```python
from build123d import *

# Parameters (mm, degrees)
SKETCH_1_W                         = 72
SKETCH_1_H                         = 40
EXTRUDE_1_DEPTH                    = 2
SKETCH_2_R                         = 7
CUT_EXTRUDE_1_DEPTH                = 3
FILLET_1_R                         = 3
SKETCH_5_R                         = 1.75
CUT_EXTRUDE_4_DEPTH                = 3
PATTERN_LINEAR_1_COUNT             = 2
PATTERN_LINEAR_1_PITCH             = 65
PATTERN_LINEAR_1_COUNT_DIR2        = 2
PATTERN_LINEAR_1_PITCH_DIR2        = 24
SKETCH_7_R                         = 2
SKETCH_7_R_2                       = 0.85
EXTRUDE_2_DEPTH                    = 3
SKETCH_8_R                         = 0.85
CUT_EXTRUDE_6_DEPTH                = 6
FILLET_3_R                         = 1
CHAMFER_1_SIZE                     = 0.6
PATTERN_LINEAR_2_COUNT             = 2
PATTERN_LINEAR_2_PITCH             = 12.5
PATTERN_LINEAR_2_COUNT_DIR2        = 2
PATTERN_LINEAR_2_PITCH_DIR2        = 21
FILLET_3_OF_PATTERN_LINEAR_2_R     = 1
CHAMFER_1_OF_PATTERN_LINEAR_2_SIZE = 0.6
CHAMFER_2_SIZE                     = 0.3


with BuildPart() as part:
    # Эскиз1 → Бобышка-Вытянуть1 (new body)
    with BuildSketch(Plane.XY):
        Rectangle(SKETCH_1_W, SKETCH_1_H)
    extrude(amount=EXTRUDE_1_DEPTH)

    # Эскиз2 → Вырез-Вытянуть1 (cut, through all)
    with BuildSketch(Plane.XY.offset(2)):
        Circle(SKETCH_2_R)
    extrude(amount=-CUT_EXTRUDE_1_DEPTH, mode=Mode.SUBTRACT)

    # Скругление1
    fillet_1_edges = [part.edges().sort_by_distance(p)[0] for p in [
        (36, -20, 1),
        (-36, -20, 1),
        (-36, 20, 1),
        (36, 20, 1),
    ]]
    fillet(fillet_1_edges, radius=FILLET_1_R)

    # Эскиз5 → Вырез-Вытянуть4 (cut, through all)
    with BuildSketch(Plane.XY.offset(2)):
        with Locations((-32.5, -12)):
            Circle(SKETCH_5_R)
    cut_extrude_4 = extrude(amount=-CUT_EXTRUDE_4_DEPTH, mode=Mode.SUBTRACT)

    # Линейный массив1: Cut-Extrude 4 2 × 2
    with Locations(*[(i * PATTERN_LINEAR_1_PITCH, j * PATTERN_LINEAR_1_PITCH_DIR2, 0) for i in range(PATTERN_LINEAR_1_COUNT) for j in range(PATTERN_LINEAR_1_COUNT_DIR2) if (i, j) != (0, 0)]):
        add(cut_extrude_4, mode=Mode.SUBTRACT)

    # Эскиз7 → Бобышка-Вытянуть2 (add)
    with BuildSketch(Plane(origin=(0, 0, 0), x_dir=(-1, 0, 0), z_dir=(0, 0, -1))):
        with Locations((-10.5, 0.4)):
            Circle(SKETCH_7_R)
        with Locations((-10.5, 0.4)):
            Circle(SKETCH_7_R_2, mode=Mode.SUBTRACT)
    extrude_2 = extrude(amount=EXTRUDE_2_DEPTH)

    # Эскиз8 → Вырез-Вытянуть6 (cut)
    with BuildSketch(Plane(origin=(0, 0, 0), x_dir=(-1, 0, 0), z_dir=(0, 0, -1))):
        with Locations((-10.5, 0.4)):
            Circle(SKETCH_8_R)
    cut_extrude_6 = extrude(amount=-CUT_EXTRUDE_6_DEPTH, mode=Mode.SUBTRACT)

    # Скругление3
    fillet_3_edges = [part.edges().sort_by_distance(p)[0] for p in [
        (12.5, 0.4, 0),
    ]]
    fillet(fillet_3_edges, radius=FILLET_3_R)

    # Фаска1
    chamfer_1_edges = [part.edges().sort_by_distance(p)[0] for p in [
        (11.35, 0.4, -3),
    ]]
    chamfer(chamfer_1_edges, length=CHAMFER_1_SIZE)

    # Линейный массив2: Бобышка-Вытянуть2, Cut-Extrude 6 2 × 2
    with Locations(*[(-j * PATTERN_LINEAR_2_PITCH_DIR2, -i * PATTERN_LINEAR_2_PITCH, 0) for i in range(PATTERN_LINEAR_2_COUNT) for j in range(PATTERN_LINEAR_2_COUNT_DIR2) if (i, j) != (0, 0)]):
        add(extrude_2)
        add(cut_extrude_6, mode=Mode.SUBTRACT)

    # Скругление3 of Линейный массив2
    fillet_3_of_pattern_linear_2_edges = [part.edges().sort_by_distance(p)[0] for p in [
        (-8.5, 0.4, 0),
        (12.5, -12.1, 0),
        (-8.5, -12.1, 0),
    ]]
    fillet(fillet_3_of_pattern_linear_2_edges, radius=FILLET_3_OF_PATTERN_LINEAR_2_R)

    # Фаска1 of Линейный массив2
    chamfer_1_of_pattern_linear_2_edges = [part.edges().sort_by_distance(p)[0] for p in [
        (-9.65, 0.4, -3),
        (11.35, -12.1, -3),
        (-9.65, -12.1, -3),
    ]]
    chamfer(chamfer_1_of_pattern_linear_2_edges, length=CHAMFER_1_OF_PATTERN_LINEAR_2_SIZE)

    # Фаска2
    chamfer_2_edges = [part.edges().sort_by_distance(p)[0] for p in [
        (11.35, -12.1, 2),
        (-9.65, -12.1, 2),
        (-7, 0, 2),
        (-36, 0, 2),
        (0, 20, 2),
        (36, 0, 2),
        (0, -20, 2),
        (35.121320344, 19.121320344, 2),
        (35.121320344, -19.121320344, 2),
        (-35.121320344, -19.121320344, 2),
        (-35.121320344, 19.121320344, 2),
        (-34.25, -12, 2),
        (30.75, -12, 2),
        (-34.25, 12, 2),
        (30.75, 12, 2),
        (11.35, 0.4, 2),
        (-9.65, 0.4, 2),
    ]]
    chamfer(chamfer_2_edges, length=CHAMFER_2_SIZE)


solid = part.part
```
CAD build for the part. Positions are in the model's coordinates, mm. Round coordinates to 2 decimals unless told otherwise and drop trailing zeros. Write each loop counter-clockwise with the first axis right and the second up, starting at its lowest first coordinate (ties: lowest second). Pieces come first, ordered by that corner, then holes. Notation, with made-up numbers: (-33.75, 20) -> (18.25, 20) arc R7 cw to (18.25, 25) -> close; hole circle Ø9 at (-38.5, -3). An arc over 180 degrees is marked (long way). Answer in a Markdown table with one row per item. Add a question column.
Item 1: Mould opens along X. For faces 1 (the face through (35.1, 19.14, 0.86)), 2 (the face through (0, -20, 1)), 3 (the face through (10.934, -14.052, -1.986)) say: pulls with the +X half, pulls with the -X half, needs draft (parallel to the pull), parting line crosses it, or undercut.
Item 2: Drop flat-ended pins along their axis: pin 1 Ø1.5 at (x, z) = (28, -1) entering from +Y; pin 2 Ø5.5 at (x, y) = (32.5, -12) entering from -Z; pin 3 Ø4 at (x, y) = (-32.5, 12) entering from +Z; pin 4 Ø2 at (x, y) = (-10.5, -12.1) entering from +Z. Give the stop position or say it passes through.
Item 3: Saw through at B-B, the plane x = 0. Write the cut outline in (y, z).
Item 4: Saw through at D-D, the plane y = 8.5. Write the cut outline in (x, z), then the cut area to 3 significant figures.
Item 5: Drill centre lines: line 1 (Y direction, x = 10.5, z = -1.45); line 2 (Y direction, x = -10.5, z = 0.8); line 3 (X direction, y = -12, z = -2.15). Where is each one in solid material? Low to high. Write a range as from..to.
Item 6: Saw through at A-A, the plane z = 1. Count the separate pieces of the cut face and the enclosed holes in it, then the cut area to 3 significant figures.
Findings below:
| question | item | result |
|---|---|---|
| 1 | face 1 | pulls with the +X half |
| 1 | face 2 | needs draft |
| 1 | face 3 | undercut |
| 2 | pin 1 | passes through |
| 2 | pin 2 | stops at z = 0 |
| 2 | pin 3 | stops at z = 1.95 |
| 2 | pin 4 | stops at z = 1.85 |
| 3 | outline | (-20, 0) -> (-7, 0) -> (-7, 1.7) -> (-7.3, 2) -> (-19.7, 2) -> (-20, 1.7) -> close; (7, 0) -> (20, 0) -> (20, 1.7) -> (19.7, 2) -> (7.3, 2) -> (7, 1.7) -> close |
| 4 | outline | (-36, 0) -> (36, 0) -> (36, 1.7) -> (35.7, 2) -> (-35.7, 2) -> (-36, 1.7) -> close |
| 4 | area | 144 mm^2 |
| 5 | line 1 | y = -14.1..-12.95, -11.25..-10.1, -1.6..-0.45, 1.25..2.4 |
| 5 | line 2 | y = -20..-12.95, -11.25..-0.45, 1.25..20 |
| 5 | line 3 | x = -12.5..-11.34, -9.66..-8.5, 8.5..9.66, 11.34..12.5 |
| 6 | separate pieces | 1 |
| 6 | enclosed holes | 9 |
| 6 | area | 2,670 mm^2 |
